```python
from build123d import *

# Parameters (mm, degrees)
SKETCH1_W             = 124
SKETCH1_H             = 46
BOSS_EXTRUDE1_DEPTH   = 80
SKETCH2_W             = 120
SKETCH2_H             = 44
CUT_EXTRUDE1_DEPTH    = 78
SKETCH3_R             = 18
CUT_EXTRUDE2_DEPTH    = 78
SKETCH4_W             = 35.964383321
SKETCH4_H             = 30.131782619
CUT_EXTRUDE3_DEPTH    = 78
FILLET1_R             = 1
FILLET2_R             = 1
FILLET3_R             = 3
F_3_0MM_DOWEL_HOLE1_D = 3


with BuildPart() as part:
    # Sketch1 → Boss-Extrude1 (new body)
    with BuildSketch(Plane.XY):
        with Locations((62, 23)):
            Rectangle(SKETCH1_W, SKETCH1_H)
    extrude(amount=BOSS_EXTRUDE1_DEPTH)

    # Sketch2 → Cut-Extrude1 (cut)
    with BuildSketch(Plane(origin=(0, 0, 0), x_dir=(-1, 0, 0), z_dir=(0, 0, -1))):
        with Locations((-62, 22)):
            Rectangle(SKETCH2_W, SKETCH2_H)
    extrude(amount=-CUT_EXTRUDE1_DEPTH, mode=Mode.SUBTRACT)

    # Sketch3 → Cut-Extrude2 (cut)
    with BuildSketch(Plane(origin=(0, 46, 0), x_dir=(1, 0, 0), z_dir=(0, 1, 0))):
        with Locations(Location((62, -29, 0), (0, 0, 270))):
            Circle(SKETCH3_R)
    extrude(amount=-CUT_EXTRUDE2_DEPTH, mode=Mode.SUBTRACT)

    # Sketch4 → Cut-Extrude3 (cut)
    with BuildSketch(Plane(origin=(0, 46, 0), x_dir=(1, 0, 0), z_dir=(0, 1, 0))):
        with Locations((61.98219166, -15.06589131)):
            Rectangle(SKETCH4_W, SKETCH4_H)
    extrude(amount=-CUT_EXTRUDE3_DEPTH, mode=Mode.SUBTRACT)

    # Fillet1
    fillet1_edges = [part.edges().sort_by_distance(p)[0] for p in [
        (62, 44, 78),
        (2, 22, 78),
        (2, 44, 39),
    ]]
    fillet(fillet1_edges, radius=FILLET1_R)

    # Fillet2
    fillet2_edges = [part.edges().sort_by_distance(p)[0] for p in [
        (122, 21.5, 78),
        (122, 44, 38.5),
        (122, 43.707106781, 77.707106781),
    ]]
    fillet(fillet2_edges, radius=FILLET2_R)

    # Fillet3
    fillet3_edges = [part.edges().sort_by_distance(p)[0] for p in [
        (124, 23, 80),
        (62, 46, 80),
        (0, 23, 80),
        (0, 46, 40),
        (124, 46, 40),
    ]]
    fillet(fillet3_edges, radius=FILLET3_R)

    # Ø3.0mm Dowel Hole1 (through all)
    with Locations(Plane(origin=(13, 12.5, 80), x_dir=(1, 0, 0), z_dir=(0, 0, 1))):
        with Locations((0, 0), (98, 0)):
            Hole(F_3_0MM_DOWEL_HOLE1_D / 2)


solid = part.part
```
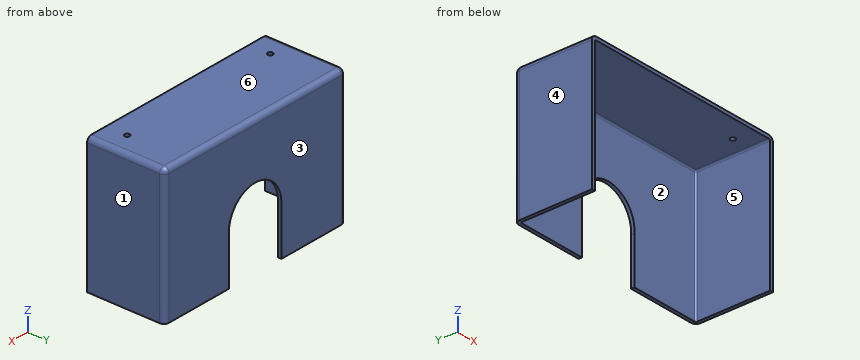
The model under review builds one solid part; all positions refer to its coordinate system, in mm. Face numbers are marked on the shaded views. A direction names the side the tool comes from. Round coordinates to 2 decimals unless told otherwise and drop trailing zeros. Order: outer loops, then holes, each group sorted by start corner. A loop starts at its lowest first (then second) coordinate and runs counter-clockwise, first axis right, second up. Notation, with made-up numbers: (-4.75, 16.25) -> (9.25, 16.25) arc R21 cw to (9.25, 39.25) -> close; hole circle Ø10 at (89, 9.25). An arc over 180 degrees is marked (long way). Use a Markdown table: item, result.
Q1. Clearance check with flat-ended pins moving along their axes: P1, Ø1.6, axis at y = 45.5, z = 10, coming from the -X side; P2, Ø1.6, axis at y = 45, z = 9, coming from the +X side; P3, Ø6, axis at x = 94.5, y = 27.5, coming from the -Z side. State where each tip first meets the part, or that it passes through.
Values:
| item | result |
|---|---|
| P1 | stops at x = 0.53 |
| P2 | stops at x = 123.75 |
| P3 | stops at z = 78 |
Q2. We need section A-A on z = 7. Write out the cut boundary in (x, y), then the cut area to 3 significant figures.
Values:
| item | result |
|---|---|
| outline | (0, 0) -> (2, 0) -> (2, 43) arc R1 cw to (3, 44) -> (44, 44) -> (44, 46) -> (3, 46) arc R3 ccw to (0, 43) -> close; (79.96, 44) -> (121, 44) arc R1 cw to (122, 43) -> (122, 0) -> (124, 0) -> (124, 43) arc R3 ccw to (121, 46) -> (79.96, 46) -> close |
| area | 349 mm^2 |
Q3. We need section B-B on y = 12.5. Write out the cut boundary in (x, z), then the cut area to 3 significant figures.
Values:
| item | result |
|---|---|
| outline | (0, 0) -> (2, 0) -> (2, 77) arc R1 cw to (3, 78) -> (11.5, 78) -> (11.5, 80) -> (3, 80) arc R3 ccw to (0, 77) -> close; (14.5, 78) -> (109.5, 78) -> (109.5, 80) -> (14.5, 80) -> close; (112.5, 78) -> (121, 78) arc R1 cw to (122, 77) -> (122, 0) -> (124, 0) -> (124, 77) arc R3 ccw to (121, 80) -> (112.5, 80) -> close |
| area | 545 mm^2 |
Q4. We need section D-D on x = 62. Write out the cut boundary in (y, z).
Values:
| item | result |
|---|---|
| outline | (0, 78) -> (43, 78) arc R1 cw to (44, 77) -> (44, 47) -> (46, 47) -> (46, 77) arc R3 ccw to (43, 80) -> (0, 80) -> close |
Q5. Tool access review of the marked faces 5 and 6: name each direction out of +Z, -Z, +X, -X, +Y, -Y from which nothing blocks a thin tool from reaching the whole face with its end or side.
Values:
| item | result |
|---|---|
| face 5 | -Z, -Y |
| face 6 | +Z, +X, -X, +Y, -Y |
Q6. Mouldability with a two-part tool opening along X and no side actions: class the marked faces 1, 2, 3 and 4 as +X half, -X half, draft (parallel to the pull), parting line (faces both ways), or undercut.
Values:
| item | result |
|---|---|
| face 1 | +X half |
| face 2 | undercut |
| face 3 | draft |
| face 4 | -X half |
Q7. For line 1 (X direction, y = 13.5, z = 56.5); line 2 (X direction, y = 12, z = 79); line 3 (Y direction, x = 74, z = 60.5), list the stretches that pass through material, from the lowest coordinate up.
Values:
| item | result |
|---|---|
| line 1 | x = 0 to 2, 122 to 124 |
| line 2 | x = 0.76 to 11.59, 14.41 to 109.59, 112.41 to 123.24 |
| line 3 | y = 44 to 46 |
Q8. We need section C-C on x = 13. Write out the cut boundary in (y, z).
Values:
| item | result |
|---|---|
| outline | (0, 78) -> (11, 78) -> (11, 80) -> (0, 80) -> close; (14, 78) -> (43, 78) arc R1 cw to (44, 77) -> (44, 0) -> (46, 0) -> (46, 77) arc R3 ccw to (43, 80) -> (14, 80) -> close |
